```python
from build123d import *

# Parameters (mm, degrees)
SKETCH_7_W               = 400
SKETCH_7_H               = 400
EXTRUDE_1_DEPTH          = 3
SKETCH_8_W               = 380
SKETCH_8_H               = 2
EXTRUDE_2_DEPTH          = 140
SKETCH_9_W               = 2
SKETCH_9_H               = 382
EXTRUDE_3_DEPTH          = 140
PATTERN_LINEAR_1_COUNT   = 12
PATTERN_LINEAR_1_PITCH   = 30
PATTERN_LINEAR_3_COUNT   = 12
PATTERN_LINEAR_3_PITCH   = 30
SKETCH_11_W              = 400
SKETCH_11_H              = 400
CUT_EXTRUDE_1_DEPTH      = 3
CUT_EXTRUDE_2_DEPTH      = 570.034269618
CUT_EXTRUDE_2_DEPTH_BACK = 570.034269618
SKETCH_12_R              = 300
SKETCH_12_R_2            = 90
SKETCH_13_R              = 92.5
SKETCH_13_R_2            = 89.5
EXTRUDE_8_DEPTH          = 140


with BuildPart() as part:
    # 草图7 → 凸台-拉伸1 (new body)
    with BuildSketch(Plane.XY):
        with Locations((200, 200)):
            Rectangle(SKETCH_7_W, SKETCH_7_H)
    extrude(amount=EXTRUDE_1_DEPTH)

    # 草图8 → 凸台-拉伸2 (add)
    with BuildSketch(Plane.XY.offset(3)):
        with Locations((200, 389)):
            Rectangle(SKETCH_8_W, SKETCH_8_H)
    extrude_2 = extrude(amount=EXTRUDE_2_DEPTH)

    # 草图9 → 凸台-拉伸3 (add)
    with BuildSketch(Plane.XY.offset(3)):
        with Locations((11, 199)):
            Rectangle(SKETCH_9_W, SKETCH_9_H)
    extrude_3 = extrude(amount=EXTRUDE_3_DEPTH)

    # 阵列(线性)1: 凸台-拉伸3 ×12
    with Locations(*[(i * PATTERN_LINEAR_1_PITCH, 0, 0) for i in range(1, PATTERN_LINEAR_1_COUNT)]):
        add(extrude_3)

    # 阵列(线性)3: 凸台-拉伸2 ×12
    with Locations(*[(0, -i * PATTERN_LINEAR_3_PITCH, 0) for i in range(1, PATTERN_LINEAR_3_COUNT)]):
        add(extrude_2)

    # 草图11 → 切除-拉伸1 (cut)
    with BuildSketch(Plane(origin=(0, 0, 0), x_dir=(-1, 0, 0), z_dir=(0, 0, -1))):
        with Locations((-200, 200)):
            Rectangle(SKETCH_11_W, SKETCH_11_H)
    extrude(amount=-CUT_EXTRUDE_1_DEPTH, mode=Mode.SUBTRACT)

    # 草图12 → 切除-拉伸2 (cut, two sides: drawn at the far end of the back side and taken through both)
    with BuildSketch(Plane(origin=(0, 0, 3), x_dir=(-1, 0, 0), z_dir=(0, 0, -1)).offset(-CUT_EXTRUDE_2_DEPTH_BACK)):
        with Locations((-191, 208.958405787)):
            Circle(SKETCH_12_R)
        with Locations((-191, 208.958405787)):
            Circle(SKETCH_12_R_2, mode=Mode.SUBTRACT)
    extrude(amount=CUT_EXTRUDE_2_DEPTH + CUT_EXTRUDE_2_DEPTH_BACK, mode=Mode.SUBTRACT)

    # 草图13 → 凸台-拉伸8 (add)
    with BuildSketch(Plane(origin=(0, 0, 3), x_dir=(-1, 0, 0), z_dir=(0, 0, -1))):
        with Locations((-191, 209)):
            Circle(SKETCH_13_R)
        with Locations((-191, 209)):
            Circle(SKETCH_13_R_2, mode=Mode.SUBTRACT)
    extrude(amount=-EXTRUDE_8_DEPTH)


solid = part.part
```
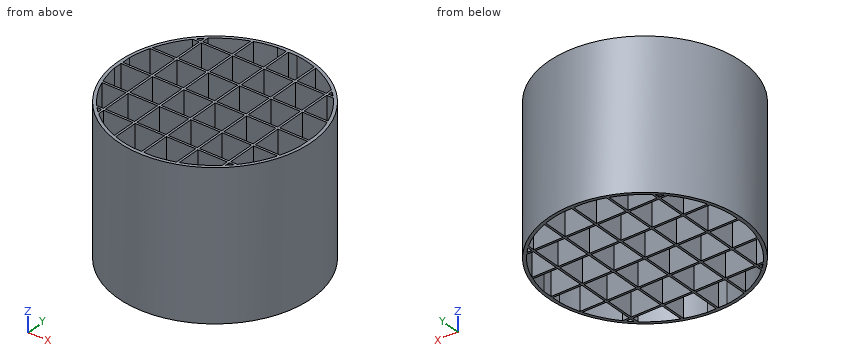
Part model, mm, in its own coordinate system. Round coordinates to 2 decimals unless told otherwise and drop trailing zeros. Order: outer loops, then holes, each group sorted by start corner. A loop starts at its lowest first (then second) coordinate and runs counter-clockwise, first axis right, second up. Notation, with made-up numbers: M 85,33 L 129,33 A5 ccw 129,39 Z; hole C -36,26 d1. An arc over 180 degrees is marked long. Answer in a Markdown table with one row per item. Add a question column.
Q1. Wall check: L1, parallel to X at y = 135.5, z = 31; L2, parallel to X at y = 130, z = 44.5; L3, parallel to Y at x = 122.5, z = 98.5. Give the ranges that are in metal, low to high. Write a range as from..to.
Q2. Pin check, flat tips, straight feed: pin 1 (1.5 mm diameter, centred on y = 195.5, z = 46.5, fed in from +X); pin 2 (22.5 mm diameter, centred on y = 277, z = 64, fed in from +X); pin 3 (12 mm diameter, centred on y = 231, z = 79, fed in from -X). Stop position of each tip, or through.
Q3. Cut at D-D on z = 53. Give the number of separate pieces and of enclosed holes in the cut face, and give its area (3 significant figures).
Q4. Cut at A-A on y = 185. Give the cut face in (x, z), and give its area (3 significant figures).
Q5. Cut at C-C on x = 115. Give the cut face in (y, z).
Q6. Cut at B-B on x = 232. Give the cut face in (y, z).
Established:
| question | item | result |
|---|---|---|
| 1 | L1 | x = 134.84..139.93, 160..162, 190..192, 220..222, 242.07..247.16 |
| 1 | L2 | x = 142.88..148.94, 160..162, 190..192, 220..222, 233.06..239.12 |
| 1 | L3 | y = 146.84..151.4, 178..180, 208..210, 238..240, 266.6..271.16 |
| 2 | pin 1 | stops at x = 282.62 |
| 2 | pin 2 | stops at x = 264.05 |
| 2 | pin 3 | stops at x = 99.89 |
| 3 | separate pieces | 1 |
| 3 | enclosed holes | 36 |
| 3 | area | 4,760 mm2 |
| 4 | outline | M 101.67,3 L 104.78,3 L 104.78,143 L 101.67,143 Z; M 130,3 L 132,3 L 132,143 L 130,143 Z; M 160,3 L 162,3 L 162,143 L 160,143 Z; M 190,3 L 192,3 L 192,143 L 190,143 Z; M 220,3 L 222,3 L 222,143 L 220,143 Z; M 250,3 L 252,3 L 252,143 L 250,143 Z; M 277.22,3 L 280.33,3 L 280.33,143 L 277.22,143 Z |
| 4 | area | 2,270 mm2 |
| 5 | outline | M 156.27,3 L 161.73,3 L 161.73,143 L 156.27,143 Z; M 178,3 L 180,3 L 180,143 L 178,143 Z; M 208,3 L 210,3 L 210,143 L 208,143 Z; M 238,3 L 240,3 L 240,143 L 238,143 Z; M 256.27,3 L 261.73,3 L 261.73,143 L 256.27,143 Z |
| 6 | outline | M 126.08,3 L 129.44,3 L 129.44,143 L 126.08,143 Z; M 148,3 L 150,3 L 150,143 L 148,143 Z; M 178,3 L 180,3 L 180,143 L 178,143 Z; M 208,3 L 210,3 L 210,143 L 208,143 Z; M 238,3 L 240,3 L 240,143 L 238,143 Z; M 268,3 L 270,3 L 270,143 L 268,143 Z; M 288.56,3 L 291.92,3 L 291.92,143 L 288.56,143 Z |
